Could you check a few things on this model? Use its own coordinates, in mm. A direction names the side the tool comes from. Give positions to 0.01 mm unless a question says otherwise; leave off trailing zeros. Loops run counter-clockwise (first coordinate to the right, second up) from the corner with the lowest first, then second, coordinate; pieces in that order, holes last. Notation, with made-up numbers: M 42,22.5 L 70,22.5 A12 ccw 70,28.5 Z; hole C -5,73.25 d6. An arc over 180 degrees is marked long. Answer in a Markdown table with one row per item. Add a question column.
1. I need wall thicknesses on line 1 along Y through (x, z) = (-14, 3); line 2 along X through (y, z) = (-10.5, 1.75); line 3 along Y through (x, z) = (-4, 0.1). Which ranges of each line are inside material? Lowest first, please. Write a range as from..to.
2. If we section it at C-C on y = -11: List the corners of the cut face in (x, z) for me (3 decimals), then the cut area to 3 significant figures.
3. If we section it at A-A on z = 2.5: List the corners of the cut face in (x, y) for me (3 decimals).
4. Which directions (+Z, -Z, +X, -X, +Y, -Y) give clear straight access to the entire face, cutting with the end or side of a thin tool? Please do faces 1 (the flat face through (0, -14.224, 2)), 2 (the flat face through (11, 14.224, 2)), 3 (the flat face through (-11, 14.224, 2)).
5. If we section it at B-B on x = -6.5: List the corners of the cut face in (y, z) for me (3 decimals), then the cut area to 3 significant figures.
6. I'm going to push flat-ended pins straight in: pin 1 Ø1 at (y, z) = (5, 1) entering from +X; pin 2 Ø1 at (y, z) = (-0.5, 2) entering from -X. Where does each tip first touch, or does it pass through?
```python
from build123d import *

# Parameters (mm, degrees)
PAD_DEPTH = 3.175
FILLET_R  = 0.889


with BuildPart() as part:
    # Sketch → Pad (new body)
    with BuildSketch(Plane.XY):
        Polygon((-17.78, 21.336), (17.78, 21.336), (17.78, 14.224), (3.556, 14.224), (3.556, -14.224), (-3.556, -14.224), (-3.556, 14.224), (-17.78, 14.224), align=None)
    extrude(amount=PAD_DEPTH)

    # Fillet
    fillet_edges = [part.edges().sort_by_distance(p)[0] for p in [
        (-17.78, 21.336, 1.5875),
        (-17.78, 14.224, 1.5875),
        (-3.556, 14.224, 1.5875),
        (17.78, 14.224, 1.5875),
        (-3.556, -14.224, 1.5875),
        (3.556, -14.224, 1.5875),
        (17.78, 21.336, 1.5875),
        (3.556, 14.224, 1.5875),
    ]]
    fillet(fillet_edges, radius=FILLET_R)


solid = part.part
```
Results:
| question | item | result |
|---|---|---|
| 1 | line 1 | 14.22..21.34 |
| 1 | line 2 | -3.56..3.56 |
| 1 | line 3 | 14.1..21.34 |
| 2 | outline | M -3.556,0 L 3.556,0 L 3.556,3.175 L -3.556,3.175 Z |
| 2 | area | 22.6 mm2 |
| 3 | outline | M -17.78,15.113 A0.889 ccw -16.891,14.224 L -4.445,14.224 A0.889 cw -3.556,13.335 L -3.556,-13.335 A0.889 ccw -2.667,-14.224 L 2.667,-14.224 A0.889 ccw 3.556,-13.335 L 3.556,13.335 A0.889 cw 4.445,14.224 L 16.891,14.224 A0.889 ccw 17.78,15.113 L 17.78,20.447 A0.889 ccw 16.891,21.336 L -16.891,21.336 A0.889 ccw -17.78,20.447 Z |
| 4 | face 1 | +Z, -Z, +X, -X, -Y |
| 4 | face 2 | +Z, -Z, +X, -Y |
| 4 | face 3 | +Z, -Z, -X, -Y |
| 5 | outline | M 14.224,0 L 21.336,0 L 21.336,3.175 L 14.224,3.175 Z |
| 5 | area | 22.6 mm2 |
| 6 | pin 1 | x = 3.56 |
| 6 | pin 2 | x = -3.56 |
